Study the drawing (mm; zero at the part's minimum x, y, z) and answer. Coordinates: 2 decimals unless noted, no trailing zeros. Loops run counter-clockwise (first coordinate to the right, second up) from the corner with the lowest first, then second, coordinate; pieces in that order, holes last. Notation, with made-up numbers: (37.5, 54.25) - (92.5, 54.25) arc R12 cw to (92.5, 61.25) - close; hole circle Ø2 at (68, 18.5). An arc over 180 degrees is marked (long way). Put each result on its own line as item: value.
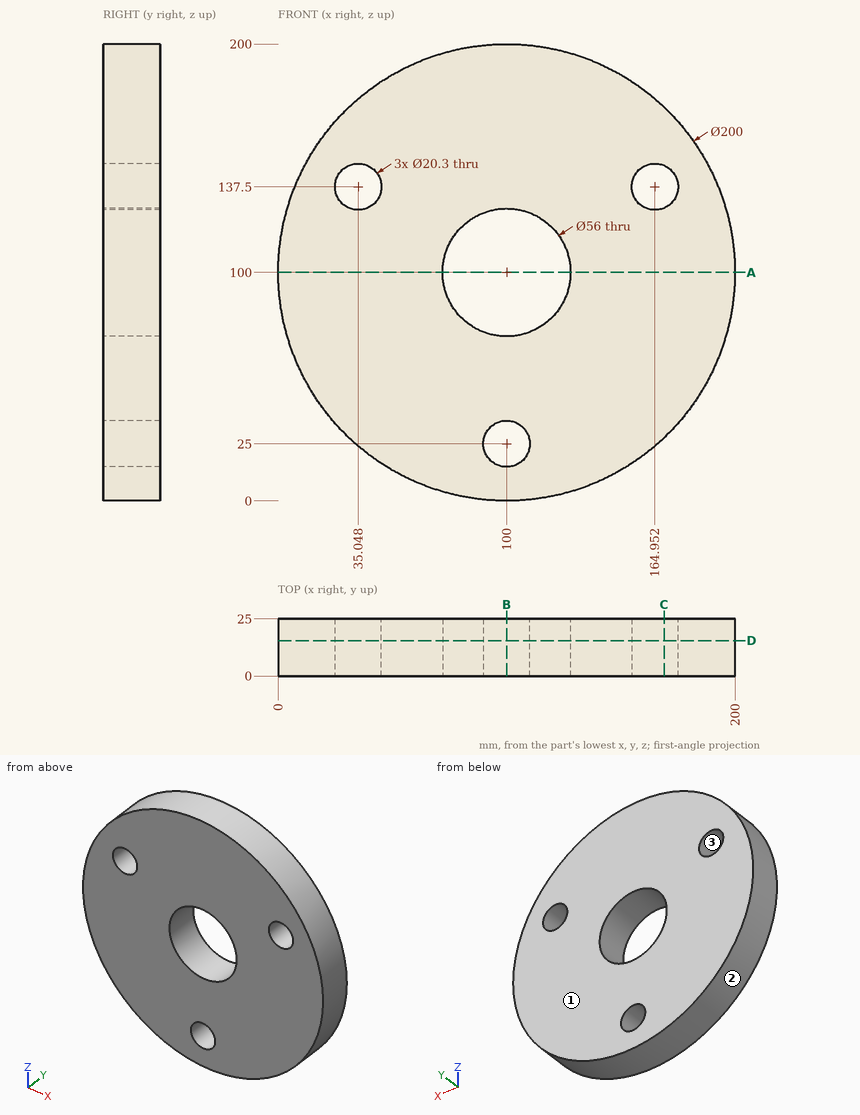
1) The part is cut by section B-B (x = 100). Give the vertices of the cut face in (y, z), and give its area (3 significant figures).
Found:
outline: (0, 0) - (25, 0) - (25, 14.85) - (0, 14.85) - close; (0, 35.15) - (25, 35.15) - (25, 72) - (0, 72) - close; (0, 128) - (25, 128) - (25, 200) - (0, 200) - close
area: 3,090 mm^2
2) Each of these flat-tipped pins is pushed along its axis until it touches: pin 1 (5 mm diameter, centred on y = 17, z = 138, fed in from -X); pin 2 (1 mm diameter, centred on x = 54, y = 17, fed in from +Z); pin 3 (10 mm diameter, centred on x = 139.5, y = 7, fed in from -Z). Where does it stop, or does it pass through?
Found:
pin 1: stops at x = 6.51
pin 2: stops at z = 189.05
pin 3: stops at z = 6.14
3) The part is cut by section C-C (x = 169). Give the vertices of the cut face in (y, z).
Found:
outline: (0, 27.62) - (25, 27.62) - (25, 128.19) - (0, 128.19) - close; (0, 146.81) - (25, 146.81) - (25, 172.38) - (0, 172.38) - close
4) For a pull along Z with two mould halves and no side action, classify the marked faces 1, 2 and 3 as pulls with the +Z half, pulls with the -Z half, needs draft (parallel to the pull), parting line crosses it, or undercut.
Found:
face 1: needs draft
face 2: parting line crosses it
face 3: undercut
5) Straight lines are drawn through the part: L1, parallel to Z at x = 100, y = 13.5; L2, parallel to X at y = 13.5, z = 100; L3, parallel to X at y = 11.75, z = 137.5. For each, find the intervals that lie inside material, in ascending order. Write a range as [from, to].
Found:
L1: z = [0, 14.85], [35.15, 72], [128, 200]
L2: x = [0, 72], [128, 200]
L3: x = [7.3, 24.9], [45.2, 154.8], [175.1, 192.7]
6) The part is cut by section D-D (y = 15.5). Give the vertices of the cut face in (x, z).
Found:
outline: circle Ø200 at (100, 100); hole circle Ø20.3 at (35.05, 137.5); hole circle Ø56 at (100, 100); hole circle Ø20.3 at (100, 25); hole circle Ø20.3 at (164.95, 137.5)
7) The part is cut by section A-A (z = 100). Give the vertices of the cut face in (x, y).
Found:
outline: (0, 0) - (72, 0) - (72, 25) - (0, 25) - close; (128, 0) - (200, 0) - (200, 25) - (128, 25) - close
